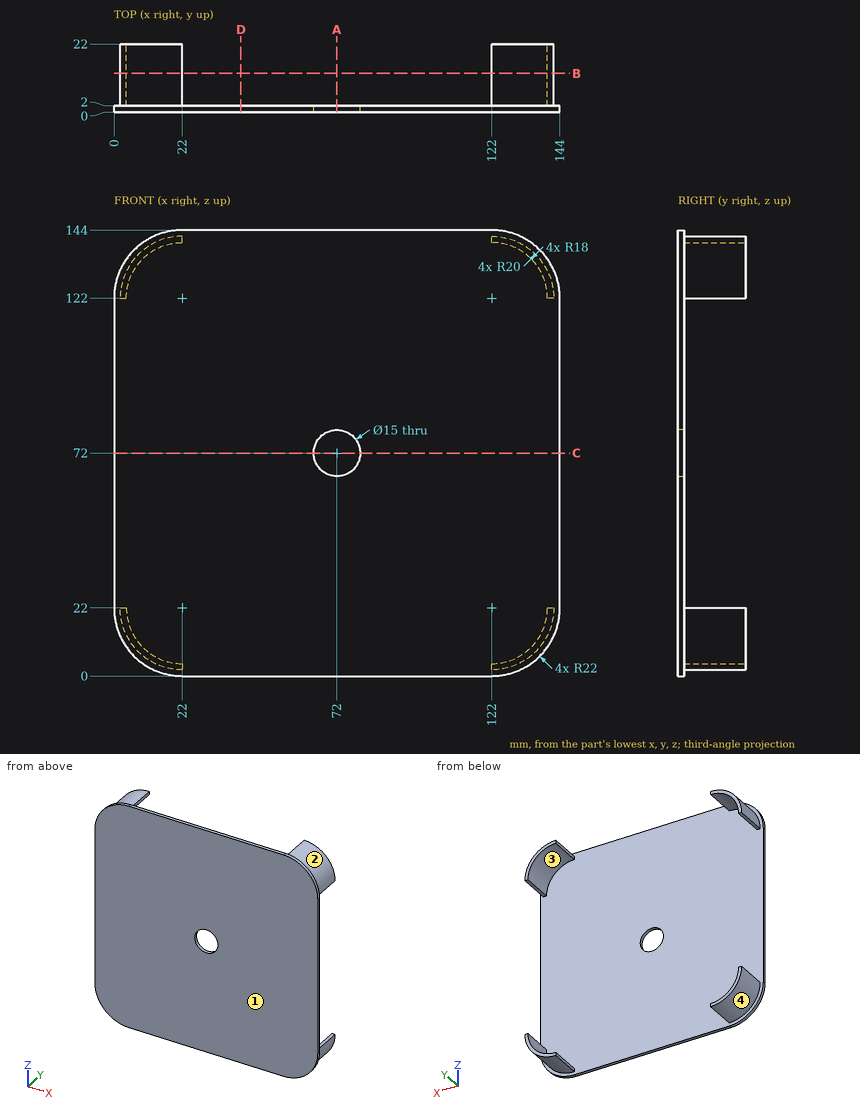
Check sheet for the drawn part. Datum: minimum x, y, z corner. Units: mm. Round coordinates to 2 decimals unless told otherwise and drop trailing zeros. Order: outer loops, then holes, each group sorted by start corner. A loop starts at its lowest first (then second) coordinate and runs counter-clockwise, first axis right, second up. Notation, with made-up numbers: M -19.5,33.5 L -15.5,33.5 A8 ccw -15.5,37.5 Z; hole C 6,-28 d8. An arc over 180 degrees is marked long. Write each question's results on one line, items separated by ' | '. Start each with the question number.
1. Material ranges on L1, parallel to X at y = 0.45, z = 72; L2, parallel to Y at x = 19, z = 92; L3, parallel to Z at x = 123, y = 2.75, recorded low to high. Write a range as from..to.
2. Cross-section at A-A on x = 72. Record the boundary of the cut face in (y, z), plus the area to 3 significant figures.
3. Draft check along X on the marked faces 1, 2, 3 and 4. Enter one of: pulls with the +X half, pulls with the -X half, needs draft (parallel to the pull), parting line crosses it, or undercut.
4. Cross-section at C-C on z = 72. Record the boundary of the cut face in (x, y), plus the area to 3 significant figures.
5. Cross-section at B-B on y = 12.5. Record the boundary of the cut face in (x, z), plus the area to 3 significant figures.
6. Go/stop test with flat-tipped pins: P1, Ø2, axis at y = 9.5, z = 3, coming from the -X side; P2, Ø12, axis at x = 46.5, y = 5.5, coming from the -Z side; P3, Ø6, axis at y = 15, z = 129, coming from the +X side; P4, Ø1, axis at y = 15.5, z = 3, coming from the +X side. Record where each tip stops, or that it passes through.
7. Cross-section at D-D on x = 41. Record the boundary of the cut face in (y, z).
Resolved:
1) L1: 0..64.5, 79.5..144 | L2: 0..2 | L3: 2.03..4.03, 139.97..141.97
2) outline: M 0,0 L 2,0 L 2,64.5 L 0,64.5 Z; M 0,79.5 L 2,79.5 L 2,144 L 0,144 Z | area: 258 mm2
3) face 1: needs draft | face 2: pulls with the +X half | face 3: undercut | face 4: pulls with the -X half
4) outline: M 0,0 L 64.5,0 L 64.5,2 L 0,2 Z; M 79.5,0 L 144,0 L 144,2 L 79.5,2 Z | area: 258 mm2
5) outline: M 2,22 A20 ccw 22,2 L 22,4 A18 cw 4,22 Z; M 2,122 L 4,122 A18 cw 22,140 L 22,142 A20 ccw Z; M 122,2 A20 ccw 142,22 L 140,22 A18 cw 122,4 Z; M 122,140 A18 cw 140,122 L 142,122 A20 ccw 122,142 Z | area: 239 mm2
6) P1: x = 13.28 | P2: z = 0 | P3: x = 141.6 | P4: x = 129.6
7) outline: M 0,0 L 2,0 L 2,144 L 0,144 Z
